Autodesk Fusion 360 part; units mm, degrees
sketch "Sketch1" plane through (0, 0, 0) normal (0, 0, 1) x (1, 0, 0)
  circle A0 centre (0, 0) radius 1.25
  line L0 (2.3094, 0) -> (1.1547, 2)
  line L1 (1.1547, 2) -> (-1.1547, 2)
  line L2 (-1.1547, 2) -> (-2.3094, 0)
  line L3 (-2.3094, 0) -> (-1.1547, -2)
  line L4 (-1.1547, -2) -> (1.1547, -2)
  line L5 (1.1547, -2) -> (2.3094, 0)
  dimension "d1" = 2.5
  dimension "d21" = 2
extrude "Extrude6" add sketch "Sketch1" along normal blind 6
extrude "Extrude7" add sketch "Sketch1" along normal blind 7 from surface at 5 contours A0
thread "Thread1" thread offset 0 thread length 10
thread "Thread2" thread offset 0 thread length 10
move_face "OffsetFaces2" offset 2 1 faces at (-1.499, 0.9014, 0)
Source: CAD feature listing. Evaluate the final solid. Frame: model axes, mm. A direction names the side the tool comes from. Round coordinates to 2 decimals unless told otherwise and drop trailing zeros. Order: outer loops, then holes, each group sorted by start corner. A loop starts at its lowest first (then second) coordinate and runs counter-clockwise, first axis right, second up. Notation, with made-up numbers: (46, 84.5) -> (57, 84.5) arc R23 cw to (57, 108.5) -> close; hole circle Ø3 at (62.5, 72.25). An arc over 180 degrees is marked (long way). One line per item, written item: value. Start each with the question number.
Q1. Section query A-A (z = 4.5). Return the cut outline in (x, y).
Q2. Section query B-B (x = 0). Return the cut outline in (y, z), plus the area to 3 significant figures.
Q3. Material intervals for probe 1 along Y at (x, z) = (0, 1.25); probe 2 along Z at (x, y) = (0.8, 0.4); probe 3 along Z at (x, y) = (-1.1, -0.75), sorted ascending.
Q4. Draft query along Y for faces 4 (the cylindrical face through (-0.27, 1.22, 8.96)), 5 (the flat face through (1.74, 0.99, 1.94)), 6 (the cylindrical face through (-0.27, 1.22, 1.45)). Return one class per face: pulls with the +Y half, pulls with the -Y half, needs draft (parallel to the pull), parting line crosses it, or undercut.
Q5. Access query for faces 1 (the flat face through (1, 1, 6)), 2 (the flat face through (0, 0, 5)), 3 (the flat face through (0, -2, 2)). Directions: +Z, -Z, +X, -X, +Y, -Y. A direction counts if a zero-diameter tool reaches every point of the face in a straight line with its end or side. Return the directions, or none.
Q6. Section query C-C (y = -0.65). Return the cut outline in (x, z), plus the area to 3 significant figures.
Q7. Section query D-D (z = 8.25). Return the cut outline in (x, y), plus the area to 3 significant figures.
Q8. Pin query (flat end, axial travel): pin 1 (0.8 mm diameter, centred on x = 0, y = 0.5, fed in from -Z). Return the tip coordinate at first contact, or that it passes through.
Findings below:
1. outline: (-2.31, 0) -> (-1.15, -2) -> (1.15, -2) -> (2.31, 0) -> (1.15, 2) -> (-1.15, 2) -> close; hole circle Ø2.5 at (0, 0)
2. outline: (-2, -2) -> (-1.25, -2) -> (-1.25, 5) -> (1.25, 5) -> (1.25, -2) -> (2, -2) -> (2, 6) -> (1.25, 6) -> (1.25, 12) -> (-1.25, 12) -> (-1.25, 6) -> (-2, 6) -> close
2. area: 29.5 mm²
3. probe 1: -2 to -1.25, 1.25 to 2
3. probe 2: 5 to 12
3. probe 3: -2 to 6
4. face 4: parting line crosses it
4. face 5: pulls with the +Y half
4. face 6: undercut
5. face 1: +Z
5. face 2: -Z
5. face 3: +Z, -Z, +X, -X, -Y
6. outline: (-1.93, -2) -> (-1.07, -2) -> (-1.07, 5) -> (1.07, 5) -> (1.07, -2) -> (1.93, -2) -> (1.93, 6) -> (1.07, 6) -> (1.07, 12) -> (-1.07, 12) -> (-1.07, 6) -> (-1.93, 6) -> close
6. area: 28.8 mm²
7. outline: circle Ø2.5 at (0, 0)
7. area: 4.91 mm²
8. pin 1: z = 5
